Could you check a few things on this model? Use its own coordinates, in mm. A direction names the side the tool comes from. Coordinates: 2 decimals unless noted, no trailing zeros. Write each loop counter-clockwise with the first axis right and the second up, starting at its lowest first coordinate (ties: lowest second). Pieces come first, ordered by that corner, then holes. Notation, with made-up numbers: (37, 37) - (52, 37) arc R14 ccw to (52, 41) - close; hole circle Ø4 at (44.25, -22). An arc over 180 degrees is marked (long way). Answer as a JSON object with one key per item and string values. Group by question number.
1) If we section it at A-A (y = 17.5): Write out the boundary of the cut face in (x, z), plus the area to 3 significant figures.
2) We'd pull the mould along X, two halves only. Please class faces 3 (the flat face through (15, 13, -6)), 4 (the flat face through (-15, 13, 6)), 5 (the conical face through (0.22, 5.62, 15.69)): released by +X, released by -X, zero draft, split by the parting line, or undercut.
3) If we section it at B-B (z = 0): Write out the boundary of the cut face in (x, y).
4) Please list where these lines run through material, in increasing order: line 1 along X through (y, z) = (18.5, -15); line 2 along Y through (x, z) = (-2.5, 0); line 3 along Z through (x, y) = (-10.25, 12).
5) If we section it at C-C (x = 9): Write out the boundary of the cut face in (y, z) (1 decimal).
6) On a 3-axis mill with a long thin cutter (end or side, diameter ignored), from which of +Z, -Z, +X, -X, +Y, -Y can I reach the whole of each face in a straight line? I mean faces 1 (the cylindrical face through (-1.258, 21.159, 18.995)), 2 (the cylindrical face through (-0.21, 21.71, 5.49)). Say none if no direction works.
7) Will this pin go through, and if not, where does the flat tip stop? pin 1 Ø8.5 at (y, z) = (17.5, 0) entering from +X.
8) If we section it at D-D (y = 31): Write out the boundary of the cut face in (x, z).
Autodesk Inventor part; units mm, degrees
ref_plane "YZ Plane" through (0, 0, 0) normal (1, 0, 0) x (0, 1, 0)
ref_plane "XZ Plane" through (0, 0, 0) normal (0, 1, 0) x (-1, 0, 0)
ref_plane "XY Plane" through (0, 0, 0) normal (0, 0, 1) x (1, 0, 0)
sketch "Esboço1" plane through (0, 0, 0) normal (0, 1, 0) x (-1, 0, 0)
  line L0 (15, -25) -> (-15, -25)
  line L1 (-15, -25) -> (-15, 25)
  line L2 (-15, 25) -> (15, 25)
  line L3 (15, 25) -> (15, -25)
  line L4 (15, -25) -> (-15, 25) construction
  line L5 (-15, -25) -> (15, 25) construction
  point P0 (0, 0)
  dimension "d0" = 30
  dimension "d1" = 50
extrude "Extrusão1" add sketch "Esboço1" along normal blind 35
sketch "Esboço3" plane through (0, 35, 0) normal (0, 1, 0) x (1, 0, 0)
  line L0 (-15, -25) -> (15, -25)
  line L1 (-15, 25) -> (-15, -25)
  point P0 (0, 0)
  point P1 (0, -15)
  dimension "d4" = 10
  dimension "d5" = 15
hole "Furo1" at (0, 35, 15) direction (0, -1, 0) diameter 8.376 depth 27.3 tip angle 118
sketch "Esboço4" plane through (0, 35, 0) normal (0, 1, 0) x (1, 0, 0)
  line L0 (15, 25) -> (-15, 25)
  line L1 (-15, 25) -> (-15, -25)
  point P0 (0, 0)
  point P1 (0, 15)
  dimension "d13" = 10
  dimension "d14" = 15
hole "Furo2" at (0, 35, -15) direction (0, -1, 0) diameter 8.376 end through all
sketch "Esboço5" plane through (15, 0, 25) normal (1, 0, 0) x (0, 0, -1)
  line L0 (0, 0) -> (0, 35)
  line L1 (0, 35) -> (50, 35)
  point P0 (25, 0)
  point P1 (25, 17.5)
  dimension "d22" = 25
  dimension "d23" = 17.5
hole "Furo3" at (15, 17.5, 0) direction (-1, 0, 0) diameter 13.835 end through all
properties part number "3D Model"
Here are the results:
{
 "1": {"outline": "(-15, -25) - (15, -25) - (15, -6.92) - (-15, -6.92) - close; (-15, 6.92) - (15, 6.92) - (15, 25) - (-15, 25) - close; hole circle Ø8.38 at (0, -15); hole circle Ø8.38 at (0, 15)", "area": "975 mm²"},
 "2": {"face 3": "released by +X", "face 4": "released by -X", "face 5": "undercut"},
 "3": {"outline": "(-15, 0) - (15, 0) - (15, 10.58) - (-15, 10.58) - close; (-15, 24.42) - (15, 24.42) - (15, 35) - (-15, 35) - close"},
 "4": {"line 1": "x = -15 to -4.19, 4.19 to 15", "line 2": "y = 0 to 10.58, 24.42 to 35", "line 3": "z = -25 to -4.2, 4.2 to 25"},
 "5": {"outline": "(0, -25) - (35, -25) - (35, 25) - (0, 25) - close; hole circle Ø13.8 at (17.5, 0)"},
 "6": {"face 1": "+Y", "face 2": "+X, -X"},
 "7": {"pin 1": "passes through"},
 "8": {"outline": "(-15, -25) - (15, -25) - (15, 25) - (-15, 25) - close; hole circle Ø8.38 at (0, -15); hole circle Ø8.38 at (0, 15)"}
}
